Source: three-view drawing plus pictorial views. Frame: mm from the lowest corner of the part. A direction names the side the tool comes from. Round coordinates to 2 decimals unless told otherwise and drop trailing zeros. Write each loop counter-clockwise with the first axis right and the second up, starting at its lowest first coordinate (ties: lowest second). Pieces come first, ordered by that corner, then holes. Notation, with made-up numbers: (-3, 20) - (52, 20) arc R23 cw to (52, 45) - close; hole circle Ø5 at (-9.5, 38). An arc over 180 degrees is marked (long way). Write each question's results on one line, items separated by ' | '.
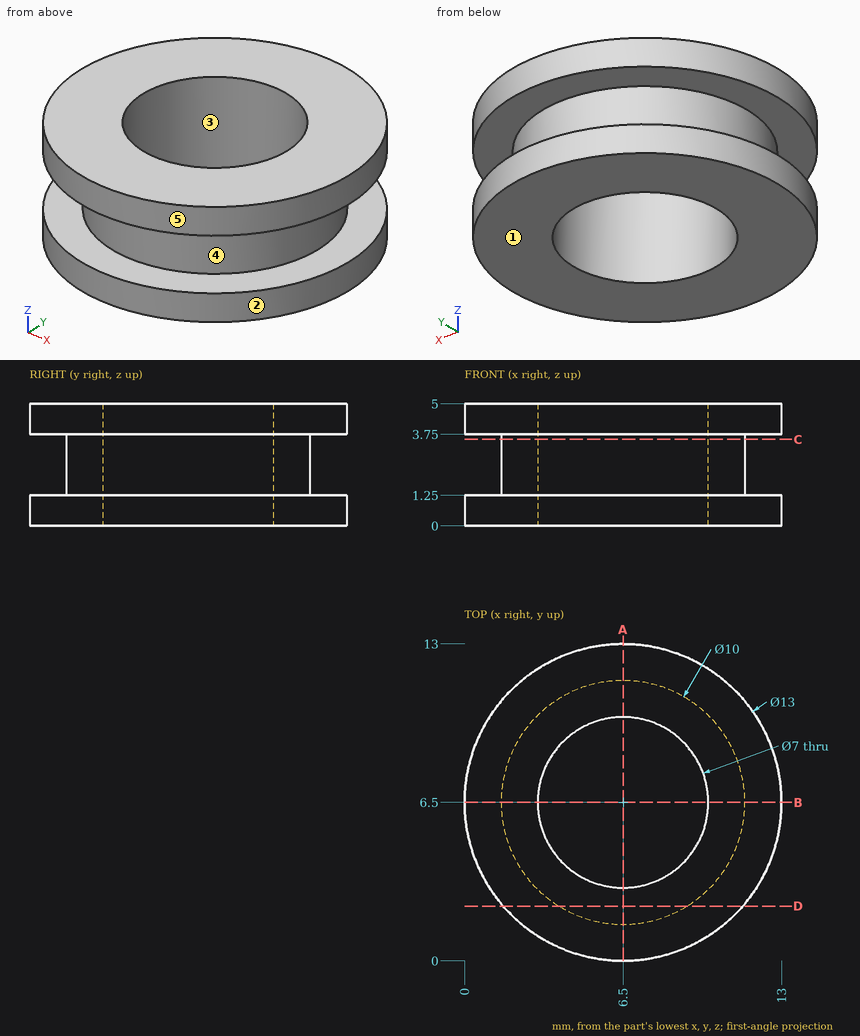
Q1. Section query D-D, the plane y = 2.25. Return loops of the section in (x, z).
Answer block:
outline: (1.58, 0) - (11.42, 0) - (11.42, 1.25) - (9.13, 1.25) - (9.13, 3.75) - (11.42, 3.75) - (11.42, 5) - (1.58, 5) - (1.58, 3.75) - (3.87, 3.75) - (3.87, 1.25) - (1.58, 1.25) - close
Q2. Ray query, line 1 along Y through (x, z) = (6.5, 2); line 2 along Y through (x, z) = (6.5, 3.8); line 3 along Z through (x, y) = (11.75, 5). Return the intervals inside material, ascending.
Answer block:
line 1: 1.5 to 3, 10 to 11.5 | line 2: 0 to 3, 10 to 13 | line 3: 0 to 1.25, 3.75 to 5
Q3. Section query C-C, the plane z = 3.55. Return loops of the section in (x, y), plus the area to 3 significant figures.
Answer block:
outline: circle Ø10 at (6.5, 6.5); hole circle Ø7 at (6.5, 6.5) | area: 40.1 mm2
Q4. Access query for the marked faces 4 and 5. Directions: +Z, -Z, +X, -X, +Y, -Y. A direction counts if a zero-diameter tool reaches every point of the face in a straight line with its end or side. Return the directions, or none.
Answer block:
face 4: none | face 5: +Z, -Z
Q5. Pin query (flat end, axial travel): pin 1 (2 mm diameter, centred on x = 10.5, z = 2, fed in from +Y); pin 2 (1.5 mm diameter, centred on x = 4.5, z = 3.5, fed in from -Y). Return the tip coordinate at first contact, or that it passes through.
Answer block:
pin 1: y = 12.08 | pin 2: y = 0.13
Q6. Mould query, pull axis X, two halves, no side actions, for the marked faces 1, 2 and 3. Classes: pulls with the +X half, pulls with the -X half, needs draft (parallel to the pull), parting line crosses it, or undercut.
Answer block:
face 1: needs draft | face 2: parting line crosses it | face 3: undercut
Q7. Section query A-A, the plane x = 6.5. Return loops of the section in (y, z).
Answer block:
outline: (0, 0) - (3, 0) - (3, 5) - (0, 5) - (0, 3.75) - (1.5, 3.75) - (1.5, 1.25) - (0, 1.25) - close; (10, 0) - (13, 0) - (13, 1.25) - (11.5, 1.25) - (11.5, 3.75) - (13, 3.75) - (13, 5) - (10, 5) - close
